The drawing under review shows one solid part. Ordinate dimensions are in mm from its lowest x, y, z. Give positions to 0.01 mm unless a question says otherwise; leave off trailing zeros. Loops run counter-clockwise (first coordinate to the right, second up) from the corner with the lowest first, then second, coordinate; pieces in that order, holes last. Notation, with made-up numbers: (48, 38) - (85, 38) arc R33 cw to (85, 66) - close; hole circle Ø1 at (16.25, -27). An arc over 180 degrees is marked (long way). Put each result on its own line as item: value. Start each with the question number.
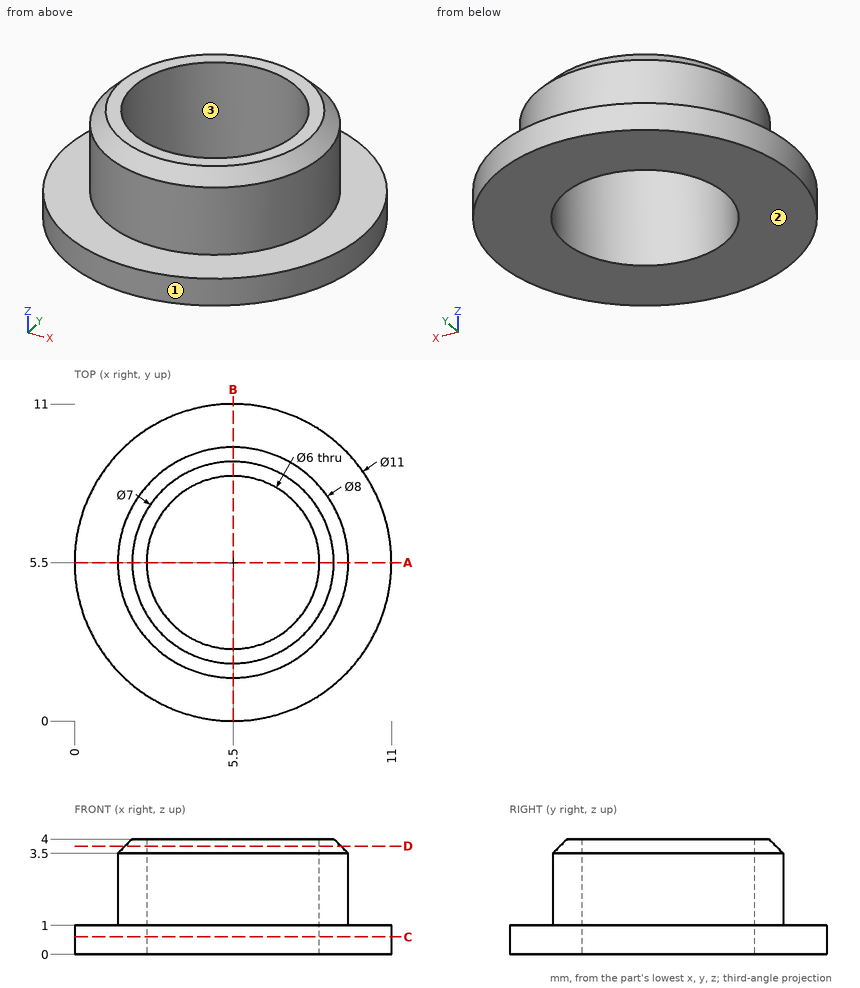
Item 1: Consider section D-D (z = 3.75). State the section outline as (x, y) points.
Item 2: Consider section A-A (y = 5.5). State the section outline as (x, z) points, plus the area to 4 significant figures.
Item 3: For P1, Ø1, axis at x = 8.5, y = 8.5, coming from the +Z side; P2, Ø1.5, axis at y = 7.5, z = 3.5, coming from the +X side; P3, Ø5, axis at x = 5.5, y = 5.5, coming from the +Z side, all flat-tipped, find the tip position at first contact; note any pin that passes through.
Item 4: For L1, parallel to Y at x = 5.5, z = 2.7; L2, parallel to Z at x = 3.5, y = 10.25; L3, parallel to Y at x = 8, z = 3.2, list the stretches that pass through material, from the lowest coordinate up. Write a range as from..to.
Item 5: Mouldability with a two-part tool opening along Y and no side actions: class the marked faces 1, 2 and 3 as pulls with the +Y half, pulls with the -Y half, needs draft (parallel to the pull), parting line crosses it, or undercut.
Item 6: Consider section C-C (z = 0.6). State the section outline as (x, y) points.
Geometry says:
1. outline: circle Ø7.5 at (5.5, 5.5); hole circle Ø6 at (5.5, 5.5)
2. outline: (0, 0) - (2.5, 0) - (2.5, 4) - (2, 4) - (1.5, 3.5) - (1.5, 1) - (0, 1) - close; (8.5, 0) - (11, 0) - (11, 1) - (9.5, 1) - (9.5, 3.5) - (9, 4) - (8.5, 4) - close
2. area: 10.75 mm2
3. P1: stops at z = 3.76
3. P2: stops at x = 9.3
3. P3: passes through
4. L1: y = 1.5..2.5, 8.5..9.5
4. L2: z = 0..1
4. L3: y = 2.38..3.84, 7.16..8.62
5. face 1: parting line crosses it
5. face 2: needs draft
5. face 3: undercut
6. outline: circle Ø11 at (5.5, 5.5); hole circle Ø6 at (5.5, 5.5)
